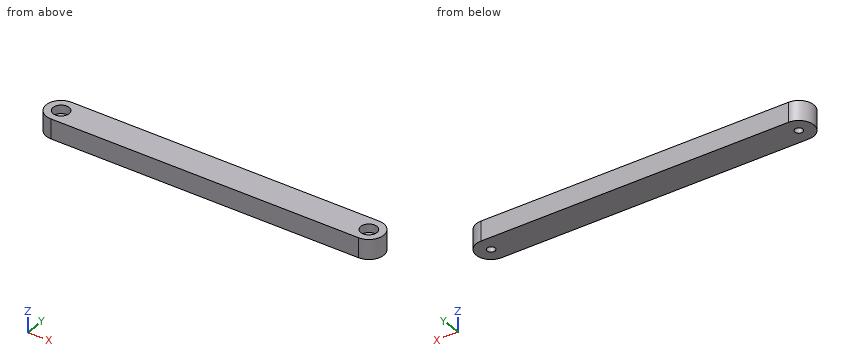
from build123d import *

# Parameters (mm, degrees)
BOSS_EXTRUDE1_DEPTH                                 = 8
CBORE_FOR_M3_HEX_SOCKET_HEAD_CAP_SCREW1_D           = 3.2
CBORE_FOR_M3_HEX_SOCKET_HEAD_CAP_SCREW1_CBORE_D     = 6.5
CBORE_FOR_M3_HEX_SOCKET_HEAD_CAP_SCREW1_CBORE_DEPTH = 3.4


with BuildPart() as part:
    # Sketch1 → Boss-Extrude1 (new body)
    with BuildSketch(Plane.XY):
        with BuildLine():
            Line((-62, 6), (62, 6))
            ThreePointArc((62, 6), (68, 0), (62, -6))
            Line((62, -6), (-62, -6))
            ThreePointArc((-62, -6), (-68, 0), (-62, 6))
        make_face()
    extrude(amount=BOSS_EXTRUDE1_DEPTH)

    # CBORE for M3 Hex Socket Head Cap Screw1 (through all)
    with Locations(Plane.XY.offset(8)):
        with Locations((-62, 0), (62, 0)):
            CounterBoreHole(CBORE_FOR_M3_HEX_SOCKET_HEAD_CAP_SCREW1_D / 2, CBORE_FOR_M3_HEX_SOCKET_HEAD_CAP_SCREW1_CBORE_D / 2, CBORE_FOR_M3_HEX_SOCKET_HEAD_CAP_SCREW1_CBORE_DEPTH)


solid = part.part
Source: CAD feature listing. Evaluate the final solid. Frame: model axes, mm. Coordinates: 2 decimals unless noted, no trailing zeros. Loops run counter-clockwise (first coordinate to the right, second up) from the corner with the lowest first, then second, coordinate; pieces in that order, holes last. Notation, with made-up numbers: (-16, 75.25) - (35, 75.25) arc R19 cw to (35, 106.25) - close; hole circle Ø11 at (40, 51). An arc over 180 degrees is marked (long way). One line per item, written item: value. Start each with the question number.
1. Ray query, L1, parallel to X at y = -0.25, z = 1.25; L2, parallel to X at y = 0.25, z = 4.75; L3, parallel to Y at x = 62, z = 7.2. Return the intervals inside material, ascending.
2. Section A-A (y = 0). Return the cut outline in (x, z), and give its area (3 significant figures).
3. Contact query for flat-ended pins moving along their axis: P1, Ø2, axis at y = -1.5, z = 4, coming from the -X side; P2, Ø2.5, axis at x = 62, y = 0, coming from the -Z side; P3, Ø4, axis at y = -3.5, z = 3.5, coming from the +X side. Output: stop coordinate, or through.
4. Section B-B (z = 3.5). Return the cut outline in (x, y).
Verdict:
1. L1: x = -67.99 to -63.58, -60.42 to 60.42, 63.58 to 67.99
1. L2: x = -67.99 to -65.24, -58.76 to 58.76, 65.24 to 67.99
1. L3: y = -6 to -3.25, 3.25 to 6
2. outline: (-68, 0) - (-63.6, 0) - (-63.6, 4.6) - (-65.25, 4.6) - (-65.25, 8) - (-68, 8) - close; (-60.4, 0) - (60.4, 0) - (60.4, 4.6) - (58.75, 4.6) - (58.75, 8) - (-58.75, 8) - (-58.75, 4.6) - (-60.4, 4.6) - close; (63.6, 0) - (68, 0) - (68, 8) - (65.25, 8) - (65.25, 4.6) - (63.6, 4.6) - close
2. area: 1,010 mm2
3. P1: stops at x = -67.98
3. P2: passes through
3. P3: stops at x = 67.81
4. outline: (-62, -6) - (62, -6) arc R6 ccw to (62, 6) - (-62, 6) arc R6 ccw to start; hole circle Ø3.2 at (-62, 0); hole circle Ø3.2 at (62, 0)
